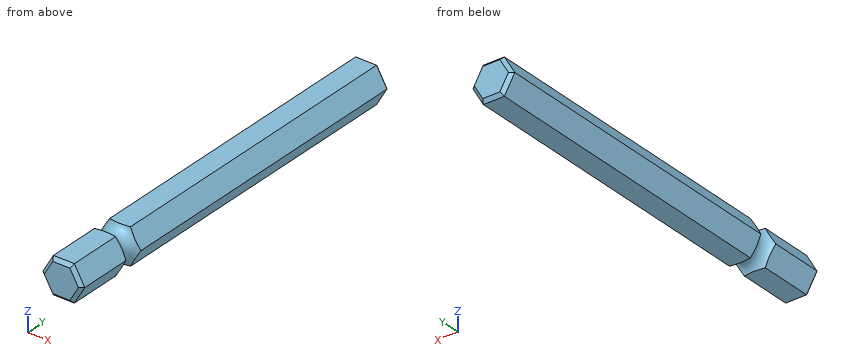
from build123d import *

# Parameters (mm, degrees)
CUT_EXTRUDE1_DEPTH      = 31.656361493
CUT_EXTRUDE1_DEPTH_BACK = 31.656361493
SKETCH5_R               = 4
CHAMFER1_SIZE           = 0.5


with BuildPart() as part:
    # Sketch2 → Revolve1 (revolve)
    with BuildSketch(Plane.XY, mode=Mode.PRIVATE) as revolve1_sk:
        with BuildLine():
            Line((-1.75, -18.5), (-1.75, 30))
            Line((-1.75, 30), (1.75, 30))
            Line((1.75, 30), (1.75, -30))
            Line((1.75, -30), (-1.75, -30))
            Line((-1.75, -30), (-1.75, -21.5))
            ThreePointArc((-1.75, -21.5), (-0.25, -20), (-1.75, -18.5))
        make_face()
    revolve(revolve1_sk.sketch.rotate(Axis((1.75, -30, 0), (0, 1, 0)), 270), axis=Axis((1.75, -30, 0), (0, 1, 0)))

    # Sketch5 → Cut-Extrude1 (cut, two sides: drawn at the far end of the back side and taken through both)
    with BuildSketch(Plane(origin=(0, 0, 0), x_dir=(1, 0, 0), z_dir=(0, 1, 0)).offset(-CUT_EXTRUDE1_DEPTH_BACK)):
        with Locations((1.75, 0)):
            Circle(SKETCH5_R)
        Polygon((4.925, 0), (3.3375, 2.749630657), (0.1625, 2.749630657), (-1.425, 0), (0.1625, -2.749630657), (3.3375, -2.749630657), align=None, mode=Mode.SUBTRACT)
    extrude(amount=CUT_EXTRUDE1_DEPTH + CUT_EXTRUDE1_DEPTH_BACK, mode=Mode.SUBTRACT)

    # Chamfer1
    chamfer1_edges = [part.edges().sort_by_distance(p)[0] for p in [
        (1.75, -30, 2.749630657),
        (4.13125, -30, 1.374815329),
        (4.13125, -30, -1.374815329),
        (1.75, -30, -2.749630657),
        (-0.63125, -30, -1.374815329),
        (-0.63125, -30, 1.374815329),
        (4.13125, 30, 1.374815329),
        (1.75, 30, 2.749630657),
        (-0.63125, 30, 1.374815329),
        (-0.63125, 30, -1.374815329),
        (1.75, 30, -2.749630657),
        (4.13125, 30, -1.374815329),
    ]]
    chamfer(chamfer1_edges, length=CHAMFER1_SIZE)


solid = part.part
Build history of the part. All positions in model axes, mm. Round coordinates to 2 decimals unless told otherwise and drop trailing zeros. Write each loop counter-clockwise with the first axis right and the second up, starting at its lowest first coordinate (ties: lowest second). Pieces come first, ordered by that corner, then holes. Notation, with made-up numbers: M -2.5,83 L 41.5,83 A28 ccw 41.5,117 Z; hole C 44.5,-2.5 d7. An arc over 180 degrees is marked long. Use CSV: the item, a comma, the result in double quotes.
1. Saw through at A-A (y = 0.5). Give the cut face in (x, z) (1 decimal), plus the area to 3 significant figures.
Reply:
outline,"M -1.4,0 L 0.2,-2.7 L 3.3,-2.7 L 4.9,0 L 3.3,2.7 L 0.2,2.7 Z"
area,"26.2 mm²"
2. Flat gauge pin, fed straight in: pin 1 (1 mm diameter, centred on y = 5, z = -1, fed in from -X). Where does the tip first touch, or does it go through?
Reply:
pin 1,"stops at x = -1.14"
3. Wall check: probe 1 along Y at (x, z) = (3, 2.5); probe 2 along Z at (x, y) = (4.75, 1); probe 3 along Y at (x, z) = (0.5, 1.85). Give the ranges that are in metal, low to high. Write a range as from..to.
Reply:
probe 1,"y = -29.75..-21.32, -18.68..29.75"
probe 2,"z = -0.3..0.3"
probe 3,"y = -30..-20.8, -19.2..30"
